Could you check a few things on this model? Use its own coordinates, in mm. A direction names the side the tool comes from. Round coordinates to 2 decimals unless told otherwise and drop trailing zeros. Loops run counter-clockwise (first coordinate to the right, second up) from the corner with the lowest first, then second, coordinate; pieces in that order, holes last. Notation, with made-up numbers: (60, -7) -> (101, -7) arc R24 ccw to (101, 31) -> close; hole circle Ø7 at (-17, 32). An arc over 180 degrees is marked (long way). One line per item, written item: value.
from build123d import *

# Parameters (mm, degrees)
CROQUIS3_W              = 688
CROQUIS3_H              = 688
SALIENTE_EXTRUIR1_DEPTH = 210
VACIADO2_T              = -0.76
CROQUIS4_W              = 160
CROQUIS4_H              = 160
CROQUIS4_W_2            = 158.247461632
CROQUIS4_H_2            = 158.247461632
SALIENTE_EXTRUIR2_DEPTH = 37


with BuildPart() as part:
    # Croquis1 → Recubrir1 section 0
    with BuildSketch(Plane(origin=(0, 0, 0), x_dir=(1, 0, 0), z_dir=(0, 1, 0))):
        with BuildLine():
            Line((-344, 344), (344, 344))
            Line((344, 344), (344, -344))
            Line((344, -344), (-344, -344))
            Line((-344, -344), (-344, 344))
        make_face()
    # Croquis2 → Recubrir1 section 1
    with BuildSketch(Plane(origin=(0, -460, 0), x_dir=(1, 0, 0), z_dir=(0, 1, 0))):
        with BuildLine():
            Line((-80, 80), (80, 80))
            Line((80, 80), (80, -80))
            Line((80, -80), (-80, -80))
            Line((-80, -80), (-80, 80))
        make_face()
    loft()

    # Croquis3 → Saliente-Extruir1 (add)
    with BuildSketch(Plane(origin=(0, 0, 0), x_dir=(1, 0, 0), z_dir=(0, 1, 0))):
        Rectangle(CROQUIS3_W, CROQUIS3_H)
    extrude(amount=SALIENTE_EXTRUIR1_DEPTH)

    # Vaciado2
    vaciado2_openings = [part.faces().sort_by_distance(p)[0] for p in [
        (0, -460, 0),
        (0, 210, 0),
    ]]
    offset(amount=VACIADO2_T, openings=vaciado2_openings, kind=Kind.INTERSECTION)

    # Croquis4 → Saliente-Extruir2 (add)
    with BuildSketch(Plane.XZ.offset(460)):
        Rectangle(CROQUIS4_W, CROQUIS4_H)
        Rectangle(CROQUIS4_W_2, CROQUIS4_H_2, mode=Mode.SUBTRACT)
    extrude(amount=SALIENTE_EXTRUIR2_DEPTH)


solid = part.part
(1) If we section it at A-A, the plane y = 31: Please give me the cut outline in (x, z).
Recorded:
outline: (-344, -344) -> (344, -344) -> (344, 344) -> (-344, 344) -> close; hole (-343.24, -343.24) -> (343.24, -343.24) -> (343.24, 343.24) -> (-343.24, 343.24) -> close
(2) Thinking about a two-plate mould opening in X: for faces 1 (the face through (79.124, -478, -1)), 2 (the face through (80, -478, -1)), 3 (the face through (-5, 104, 344)), 4 (the face through (343.24, 104, 5)), which applies, released by +X, released by -X, zero draft, split by the parting line, or undercut?
Recorded:
face 1: undercut
face 2: released by +X
face 3: zero draft
face 4: undercut
(3) If I drill on L1, parallel to X at y = 56, z = 72; L2, parallel to X at y = -208, z = 183, over which ranges is the centre line in solid material (lowest first)?
Recorded:
L1: -344 to -343.24, 343.24 to 344
L2: -224.63 to -223.75, 223.75 to 224.63
(4) For faces 5 (the face through (-1, -478, 80)), 6 (the face through (344, 104, 5)), 7 (the face through (-80, -478, -1)), 8 (the face through (-5, 104, 343.24)), 9 (the face through (-1, -478, -80)), which set-ups out of +Z, -Z, +X, -X, +Y, -Y let a thin tool reach every point of the face, with its end or its side?
Recorded:
face 5: +Z, +X, -X, -Y
face 6: +Z, -Z, +X, +Y, -Y
face 7: +Z, -Z, -X, -Y
face 8: +Y
face 9: -Z, +X, -X, -Y
(5) I'm going to push flat-ended pins straight in: pin 1 Ø5 at (x, z) = (-2, -199.5) entering from -Y; pin 2 Ø11 at (y, z) = (-471.5, -12) entering from +X; pin 3 Ø2 at (x, y) = (-156.5, -215.5) entering from +Z. Where does each tip first touch, or does it pass through?
Recorded:
pin 1: y = -256.14
pin 2: x = 80
pin 3: z = 220.9
